The listing builds one solid part. Answer for the finished solid, in the listing's coordinates (mm). A direction names the side the tool comes from. Round coordinates to 2 decimals unless told otherwise and drop trailing zeros. Order: outer loops, then holes, each group sorted by start corner. A loop starts at its lowest first (then second) coordinate and runs counter-clockwise, first axis right, second up. Notation, with made-up numbers: (-29.5, -18) -> (23.5, -18) arc R19 ccw to (23.5, -10) -> close; hole circle Ø7 at (35, 69). An arc over 180 degrees is marked (long way). Answer in a Markdown table with one row per item. Add a question column.
```python
from build123d import *

# Parameters (mm, degrees)
SKETCH1_R           = 14.8
BOSS_EXTRUDE1_DEPTH = 12
SKETCH2_R           = 16.4
BOSS_EXTRUDE2_DEPTH = 3.3
FILLET1_R           = 3.8
SKETCH3_R           = 12.2
BOSS_EXTRUDE3_DEPTH = 4
CHAMFER1_SIZE       = 0.5
CHAMFER1_SIZE2      = 12
FILLET2_R           = 0.5


with BuildPart() as part:
    # Sketch1 → Boss-Extrude1 (new body)
    with BuildSketch(Plane(origin=(0, 0, 0), x_dir=(1, 0, 0), z_dir=(0, 1, 0))):
        with Locations(Location((0, 0, 0), (0, 0, 270))):
            Circle(SKETCH1_R)
    extrude(amount=BOSS_EXTRUDE1_DEPTH)

    # Sketch2 → Boss-Extrude2 (add)
    with BuildSketch(Plane(origin=(0, 12, 0), x_dir=(1, 0, 0), z_dir=(0, 1, 0))):
        with Locations(Location((0, 0, 0), (0, 0, 270))):
            Circle(SKETCH2_R)
    extrude(amount=BOSS_EXTRUDE2_DEPTH)

    # Fillet1
    # the kernel refuses this fillet: 3.8 mm, written as the material it takes off along each edge
    with BuildSketch(Plane(origin=(0, 15.3, 0), x_dir=(0, 0, 1), z_dir=(-1, 0, 0))) as fillet1_piece_1:
        with BuildLine():
            CenterArc((12.63303836, -3.8), FILLET1_R, 7.560843177, 82.439156823)
            Line((12.63303836, 0), (12.63303836, 0.076))
            Line((12.63303836, 0.076), (16.4, 0.076))
            Line((16.4, 0.076), (16.476, 0))
            ThreePointArc((16.476, 0), (16.476, -1.65), (16.475339233, -3.29))
            Line((16.475339233, -3.29), (16.4, -3.3))
        make_face()
    revolve(axis=Axis((0, 15.3, 0), (0, 1, 0)), mode=Mode.SUBTRACT)

    # Sketch3 → Boss-Extrude3 (add)
    with BuildSketch(Plane(origin=(0, 15.3, 0), x_dir=(1, 0, 0), z_dir=(0, 1, 0))):
        with Locations(Location((0, 0, 0), (0, 0, 270))):
            Circle(SKETCH3_R)
    extrude(amount=BOSS_EXTRUDE3_DEPTH)

    # Chamfer1
    chamfer1_edges = [part.edges().sort_by_distance(p)[0] for p in [
        (0, 19.3, -12.2),
    ]]
    chamfer1_side = [part.faces().sort_by_distance(p)[0] for p in [
        (0, 17.3, -12.2),
    ]]
    chamfer(chamfer1_edges, length=CHAMFER1_SIZE, length2=CHAMFER1_SIZE2, reference=chamfer1_side[0])

    # Fillet2
    fillet2_edges = [part.edges().sort_by_distance(p)[0] for p in [
        (0, 18.8, -12.2),
    ]]
    fillet(fillet2_edges, radius=FILLET2_R)


solid = part.part
```
Item 1: The part is cut by section A-A, the plane y = 6. Give the vertices of the cut face in (x, z), and give its area (3 significant figures).
Item 2: Flat-ended cylindrical pins translate along their axes: P1, Ø1, axis at y = 11, z = -12, coming from the -X side; P2, Ø1, axis at x = 0.5, y = 3, coming from the -Z side; P3, Ø2, axis at x = -10, z = -10, coming from the -Y side; P4, Ø3, axis at x = 5.5, z = 7.5, coming from the +Y side. Find the tip coordinate at first contact, or state that the pin passes through.
Item 3: Find the intervals of material crossed by probe 1 along Y at (x, z) = (11.5, -1.5); probe 2 along Z at (x, y) = (8.5, 9); probe 3 along Y at (x, z) = (11, -9), in increasing order. Write a range as [from, to].
Item 4: A tool of negligible diameter and unlimited length cuts with its end or side. For faces 1 (the face through (-14.448, 5.916, -3.208)), 2 (the face through (0, 0, 0)), 3 (the face through (3.66, 16.79, 11.64)), from which of +Z, -Z, +X, -X, +Y, -Y can it reach the whole face along a straight path? Write none if from no direction.
Resolved:
| question | item | result |
|---|---|---|
| 1 | outline | circle Ø29.6 at (0, 0) |
| 1 | area | 688 mm2 |
| 2 | P1 | x = -9.32 |
| 2 | P2 | z = -14.8 |
| 2 | P3 | y = 0 |
| 2 | P4 | y = 18.98 |
| 3 | probe 1 | [0, 18.83] |
| 3 | probe 2 | [-12.12, 12.12] |
| 3 | probe 3 | [0, 14.96] |
| 4 | face 1 | -Y |
| 4 | face 2 | +Z, -Z, +X, -X, -Y |
| 4 | face 3 | +Y |
